```python
from build123d import *

# Parameters (mm, degrees)
SKETCH_1_W          = 38
SKETCH_1_H          = 27
SKETCH_1_R          = 1.1
SKETCH_1_R_2        = 1.6
EXTRUDE_1_DEPTH     = 3
SKETCH_2_R          = 7.5
SKETCH_2_W          = 18
SKETCH_2_H          = 19
CUT_EXTRUDE_1_DEPTH = 21.5
FILLET_1_R          = 10
CUT_EXTRUDE_2_DEPTH = 21.5
FILLET_2_R          = 2


with BuildPart() as part:
    # 草图1 → 凸台-拉伸1 (new body)
    with BuildSketch(Plane(origin=(0, 0, 0), x_dir=(1, 0, 0), z_dir=(0, 1, 0))):
        with Locations((9.5, -4)):
            Rectangle(SKETCH_1_W, SKETCH_1_H)
        with Locations(Location((7.5, -7.5, 0), (0, 0, 270))):
            Circle(SKETCH_1_R, mode=Mode.SUBTRACT)
        with Locations(Location((7.5, 7.5, 0), (0, 0, 270))):
            Circle(SKETCH_1_R, mode=Mode.SUBTRACT)
        with Locations(Location((-7.5, 7.5, 0), (0, 0, 270))):
            Circle(SKETCH_1_R, mode=Mode.SUBTRACT)
        with Locations(Location((-7.5, -7.5, 0), (0, 0, 270))):
            Circle(SKETCH_1_R, mode=Mode.SUBTRACT)
        with Locations(Location((3.5, -14.5, 0), (0, 0, 270))):
            Circle(SKETCH_1_R_2, mode=Mode.SUBTRACT)
        with Locations(Location((23.5, -14.5, 0), (0, 0, 270))):
            Circle(SKETCH_1_R_2, mode=Mode.SUBTRACT)
    extrude(amount=EXTRUDE_1_DEPTH)

    # 草图2 → 切除-拉伸1 (cut)
    with BuildSketch(Plane(origin=(0, 3, 0), x_dir=(1, 0, 0), z_dir=(0, 1, 0))):
        with Locations(Location((0, 0, 0), (0, 0, 270))):
            Circle(SKETCH_2_R)
        with Locations((19.5, 0)):
            Rectangle(SKETCH_2_W, SKETCH_2_H)
    extrude(amount=-CUT_EXTRUDE_1_DEPTH, mode=Mode.SUBTRACT)

    # 圆角1
    fillet_1_edges = [part.edges().sort_by_distance(p)[0] for p in [
        (10.5, 1.5, 9.5),
        (-9.5, 1.5, 17.5),
    ]]
    fillet(fillet_1_edges, radius=FILLET_1_R)

    # 草图3 → 切除-拉伸2 (cut)
    with BuildSketch(Plane(origin=(0, 3, 0), x_dir=(1, 0, 0), z_dir=(0, 1, 0))):
        with BuildLine():
            Line((9.5, -10.5), (17.5, -10.5))
            ThreePointArc((17.5, -10.5), (19.5, -12.5), (17.5, -14.5))
            Line((17.5, -14.5), (9.5, -14.5))
            ThreePointArc((9.5, -14.5), (7.5, -12.5), (9.5, -10.5))
        make_face()
    extrude(amount=-CUT_EXTRUDE_2_DEPTH, mode=Mode.SUBTRACT)

    # 圆角2
    fillet_2_edges = [part.edges().sort_by_distance(p)[0] for p in [
        (10.5, 1.5, -9.5),
        (28.5, 1.5, 9.5),
        (-9.5, 1.5, -9.5),
        (28.5, 1.5, 17.5),
    ]]
    fillet(fillet_2_edges, radius=FILLET_2_R)


solid = part.part
```
Check sheet for the modelled part. Datum: model origin and axes. Units: mm. A direction names the side the tool comes from. Round coordinates to 2 decimals unless told otherwise and drop trailing zeros. Loops run counter-clockwise (first coordinate to the right, second up) from the corner with the lowest first, then second, coordinate; pieces in that order, holes last. Notation, with made-up numbers: (62, 0) - (105, 0) arc R30 cw to (105, 37) - close; hole circle Ø5 at (-25.5, 65.25). An arc over 180 degrees is marked (long way). Write item = value, one per line. Start each with the question number.
Q1. Section check C-C (z = 12.5). Record the boundary of the cut face in (x, y).
Q2. Access from +Z, -Z, +X, -X, +Y, -Y to the whole of each face (thin tool, end or side, straight path). Record for faces 5 (the face through (-9.5, 1, 0)), 6 (the face through (23, 2, 9.5)), 7 (the face through (14, 2, 14.5)).
Q3. Depth check by flat-ended pin: P1, Ø0.9, axis at x = 12.5, y = 2, coming from the -Z side; P2, Ø1, axis at y = 0.5, z = 3.5, coming from the +X side. Enter the tip coordinate at first touch or a pass-through.
Q4. Section check A-A (x = 23.5). Record the boundary of the cut face in (y, z), plus the area to 3 significant figures.
Q5. Thickness scan on L1, parallel to Z at x = -5, y = 2.2; L2, parallel to X at y = 2.25, z = 0; L3, parallel to X at y = 1.75, z = 3. Record the ranges inside material, lowest first.
Q6. Release check for a two-part mould opening along X. For faces 1 (the face through (19.5, 1.5, 12.5)), 2 (the face through (0.33, 1.521, -7.493)), 3 (the face through (-6.65, 1.52, 14.49)), 4 (the face through (28.5, 1, 14)) record: pulls with the +X half, pulls with the -X half, needs draft (parallel to the pull), parting line crosses it, or undercut.
Q7. Section check B-B (y = 1.15). Count the separate pieces of the cut face and the enclosed holes in it, plus the area to 3 significant figures.
Derived:
q1.outline = (-8.16, 0) - (7.5, 0) - (7.5, 3) - (-8.16, 3) - close; (19.5, 0) - (28.5, 0) - (28.5, 3) - (19.5, 3) - close
q2.face_5 = +Z, -Z, -X, +Y, -Y
q2.face_6 = -Z, +X, +Y, -Y
q2.face_7 = +Y, -Y
q3.P1 = 4.85
q3.P2 = 11.57
q4.outline = (0, 9.5) - (3, 9.5) - (3, 12.9) - (0, 12.9) - close; (0, 16.1) - (3, 16.1) - (3, 17.5) - (0, 17.5) - close
q4.area = 14.4 mm^2
q5.L1 = -9.5 to -5.59, 5.59 to 15.85
q5.L2 = -9.5 to -7.5, 7.5 to 10.51
q5.L3 = -9.5 to -6.87, 6.87 to 11.13
q6.face_1 = undercut
q6.face_2 = undercut
q6.face_3 = pulls with the -X half
q6.face_4 = pulls with the +X half
q7.separate_pieces = 1
q7.enclosed_holes = 8
q7.area = 428 mm^2
